Build history of the part. All positions in model axes, mm. Give positions to 0.01 mm unless a question says otherwise; leave off trailing zeros. Order: outer loops, then holes, each group sorted by start corner. A loop starts at its lowest first (then second) coordinate and runs counter-clockwise, first axis right, second up. Notation, with made-up numbers: (-22, 68) -> (-14, 68) arc R20 cw to (-14, 79) -> close; hole circle Ø11 at (68.5, 0). An arc over 180 degrees is marked (long way). One line per item, written item: value. Start each with the question number.
(1) Probe line 1 (Z direction, x = 0, y = -21) (3 decimals); line 2 (X direction, y = -14, z = 1.5); line 3 (Z direction, x = -13.5, y = -57). List the from-to ranges inside material, lowest first.
(2) Two-plate mould, pull along Z, no slides. Class faces 1 (the flat face through (-62, 0, 39)), 2 (the cylindrical face through (69.653, -37.567, 21.935)), 3 (the cylindrical face through (-55.431, -37.567, -42.503)): +Z half, -Z half, draft (parallel to the pull), parting line (faces both ways), or undercut.
(3) Pin check, flat tips, straight feed: pin 1 (1.5 mm diameter, centred on x = 54.5, y = 30.5, fed in from -Z); pin 2 (1 mm diameter, centred on x = -10.5, y = 24, fed in from -Z); pin 3 (4 mm diameter, centred on x = -42, y = 13, fed in from +Z). Stop position of each tip, or through.
(4) Saw through at A-A on y = -61. Give the cut face in (x, z) (3 decimals).
```python
from build123d import *

# Parameters (mm, degrees)
SKETCH7_R           = 317.5
CUT_EXTRUDE2_DEPTH  = 279.4
SKETCH8_R           = 73.025
SKETCH8_R_2         = 69.85
BOSS_EXTRUDE1_DEPTH = 76.2


with BuildPart() as part:
    # Sketch2 → Revolve1 (revolve)
    with BuildSketch(Plane.XY):
        with BuildLine():
            Line((-76.2, 0), (-69.85, 0))
            ThreePointArc((-69.85, 0), (-46.178344337, 164.977710697), (0, 325.12))
            Line((0, 325.12), (0, 330.2))
            ThreePointArc((0, 330.2), (-50.970594074, 168.070137094), (-76.2, 0))
        make_face()
    revolve(axis=Axis((0, 330.2, 0), (0, -1, 0)))

    # Sketch7 → Cut-Extrude2 (cut)
    with BuildSketch(Plane(origin=(0, 381, 0), x_dir=(1, 0, 0), z_dir=(0, 1, 0))):
        Circle(SKETCH7_R)
    extrude(amount=-CUT_EXTRUDE2_DEPTH, mode=Mode.SUBTRACT)

    # Sketch8 → Boss-Extrude1 (add)
    with BuildSketch(Plane.XZ):
        Circle(SKETCH8_R)
        Circle(SKETCH8_R_2, mode=Mode.SUBTRACT)
    extrude(amount=BOSS_EXTRUDE1_DEPTH)


solid = part.part
```
Results below:
1. line 1: z = -73.025 to -69.85, 69.85 to 73.025
1. line 2: x = -73.01 to -69.83, 69.83 to 73.01
1. line 3: z = -71.77 to -68.53, 68.53 to 71.77
2. face 1: draft
2. face 2: parting line
2. face 3: undercut
3. pin 1: stops at z = -50.28
3. pin 2: stops at z = -73.56
3. pin 3: stops at z = 63.69
4. outline: circle Ø146.05 at (0, 0); hole circle Ø139.7 at (0, 0)
